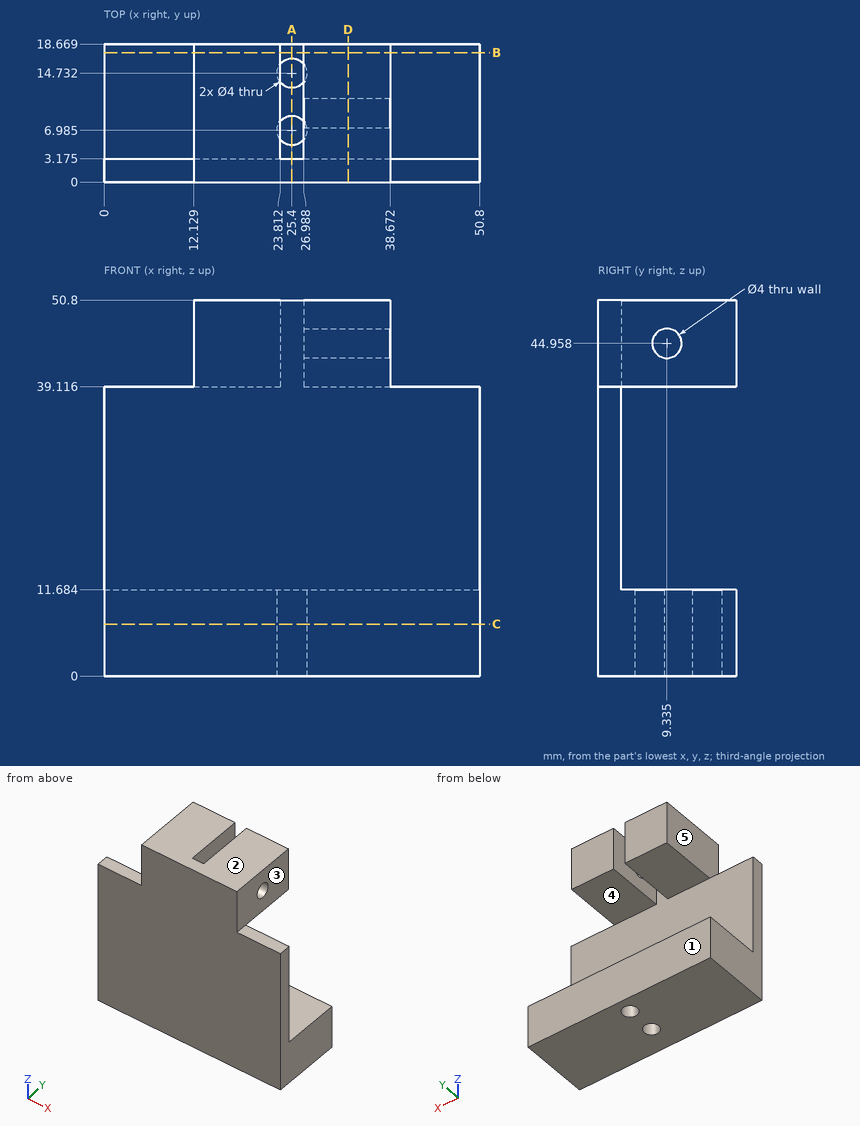
Geometry check sheet. Reference: drawing and pictorial views, mm from the part's lowest x, y, z. A direction names the side the tool comes from. Coordinates: 2 decimals unless noted, no trailing zeros. Write each loop counter-clockwise with the first axis right and the second up, starting at its lowest first coordinate (ties: lowest second). Pieces come first, ordered by that corner, then holes. Notation, with made-up numbers: (54.25, -36.75) - (87.25, -36.75) arc R7 cw to (87.25, -27.75) - close; hole circle Ø6 at (-4.5, -35). An arc over 180 degrees is marked (long way). Write item = value, one per line.
Q1. Cross-section at B-B (y = 17.5). Enter the section's corners in (x, z) (1 decimal).
Answer:
outline = (0, 0) - (50.8, 0) - (50.8, 11.7) - (0, 11.7) - close; (12.1, 39.1) - (23.8, 39.1) - (23.8, 50.8) - (12.1, 50.8) - close; (27, 39.1) - (38.7, 39.1) - (38.7, 50.8) - (27, 50.8) - close
Q2. Cross-section at D-D (x = 33). Enter the section's corners in (y, z) (1 decimal), plus the area to 3 significant figures.
Answer:
outline = (0, 0) - (18.7, 0) - (18.7, 11.7) - (3.2, 11.7) - (3.2, 39.1) - (18.7, 39.1) - (18.7, 50.8) - (0, 50.8) - close; hole circle Ø4 at (9.3, 45)
area = 511 mm²
Q3. Access from +Z, -Z, +X, -X, +Y, -Y to the whole of each face (thin tool, end or side, straight path). Record for the marked faces 1, 2, 3, 4 and 5.
Answer:
face_1 = +Z, -Z, +X, -X, +Y
face_2 = +Z, +X, -X, +Y, -Y
face_3 = +Z, +X, +Y, -Y
face_4 = +X, -X, +Y
face_5 = +Z, -X, +Y, -Y
Q4. Material ranges on L1, parallel to Y at x = 25.4, z = 6.5 (1 decimal); L2, parallel to Z at x = 16, y = 9.5 (1 decimal); L3, parallel to Z at x = 37.5, y = 7.75 (1 decimal), recorded low to high. Write a range as from..to.
Answer:
L1 = 0..5, 9..12.7, 16.7..18.7
L2 = 0..11.7, 39.1..50.8
L3 = 0..11.7, 39.1..43.7, 46.2..50.8
Q5. Cross-section at C-C (z = 7). Enter the section's corners in (x, y) (1 decimal), plus the area to 3 significant figures.
Answer:
outline = (0, 0) - (50.8, 0) - (50.8, 18.7) - (0, 18.7) - close; hole circle Ø4 at (25.4, 7); hole circle Ø4 at (25.4, 14.7)
area = 923 mm²
Q6. Go/stop test with flat-tipped pins: pin 1 Ø11.5 at (x, z) = (24, 27.5) entering from +Y (1 decimal); pin 2 Ø6 at (y, z) = (8.5, 43) entering from -X; pin 3 Ø2 at (x, z) = (44.5, 15.5) entering from -Y; pin 4 Ø3.5 at (x, y) = (44.5, 1.5) entering from +Z. Record where each tip stops, or that it passes through.
Answer:
pin_1 = 3.2
pin_2 = 12.13
pin_3 = 0
pin_4 = 39.12
Q7. Cross-section at A-A (x = 25.4). Enter the section's corners in (y, z) (1 decimal).
Answer:
outline = (0, 0) - (5, 0) - (5, 11.7) - (3.2, 11.7) - (3.2, 50.8) - (0, 50.8) - close; (9, 0) - (12.7, 0) - (12.7, 11.7) - (9, 11.7) - close; (16.7, 0) - (18.7, 0) - (18.7, 11.7) - (16.7, 11.7) - close
